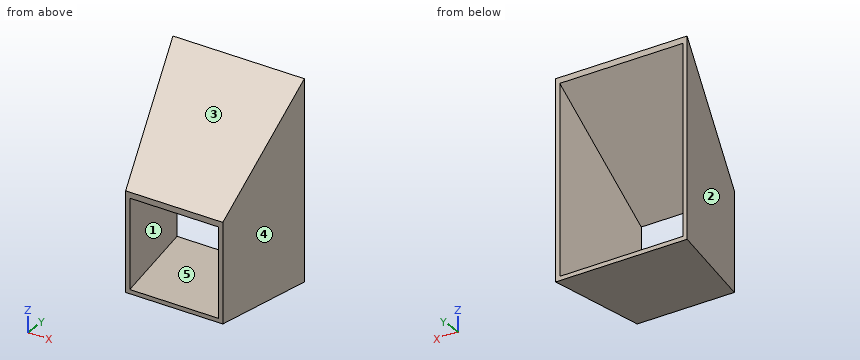
from build123d import *

# Parameters (mm, degrees)
BOSS_EXTRUDE1_DEPTH     = 120
CUT_EXTRUDE1_DEPTH      = 131.179512464
CUT_EXTRUDE1_DEPTH_BACK = 131.179512464
SHELL1_T                = -2.5


with BuildPart() as part:
    # Sketch1 → Boss-Extrude1 (new body)
    with BuildSketch(Plane.XY):
        Polygon((-40.579618843, 30), (40.579618843, 30), (30, -30), (-30, -30), align=None)
    extrude(amount=BOSS_EXTRUDE1_DEPTH)

    # Sketch2 → Cut-Extrude1 (cut, two sides: drawn at the far end of the back side and taken through both)
    with BuildSketch(Plane(origin=(0, 0, 0), x_dir=(0, 0, -1), z_dir=(1, 0, 0)).offset(-CUT_EXTRUDE1_DEPTH_BACK)):
        Polygon((-120, 30), (-120, -30), (-60, -30), align=None)
    extrude(amount=CUT_EXTRUDE1_DEPTH + CUT_EXTRUDE1_DEPTH_BACK, mode=Mode.SUBTRACT)

    # Shell1
    shell1_openings = [part.faces().sort_by_distance(p)[0] for p in [
        (0, -30, 30),
        (0, 30, 60),
    ]]
    offset(amount=SHELL1_T, openings=shell1_openings, kind=Kind.INTERSECTION)


solid = part.part
Part model, mm, in its own coordinate system. Face numbers are marked on the shaded views. A direction names the side the tool comes from. Give positions to 0.01 mm unless a question says otherwise; leave off trailing zeros. Loops run counter-clockwise (first coordinate to the right, second up) from the corner with the lowest first, then second, coordinate; pieces in that order, holes last.
(1) 3-axis set-ups, long thin cutter, end or side, ignore diameter. For the marked faces 1 and 2: which of +Z, -Z, +X, -X, +Y, -Y reach the whole face in a straight line?
Return value:
face 1: +Y
face 2: +Z, -Z, -X, -Y
(2) Drill centre lines: line 1 along Z through (x, y) = (14, -5); line 2 along Z through (x, y) = (-13, -4); line 3 along X through (y, z) = (-12.5, 27). Where is each one in solid material? Low to high.
Return value:
line 1: z = 0 to 2.5, 81.46 to 85
line 2: z = 0 to 2.5, 82.46 to 86
line 3: x = -33.09 to -30.55, 30.55 to 33.09
(3) Pin check, flat tips, straight feed: pin 1 (8 mm diameter, centred on x = -19.5, z = 25, fed in from +Y); pin 2 (1.5 mm diameter, centred on x = 3.5, z = 68, fed in from +Y); pin 3 (4 mm diameter, centred on y = -15, z = 12.5, fed in from -X); pin 4 (1.5 mm diameter, centred on y = 21, z = 38.5, fed in from +X). Stop position of each tip, or through.
Return value:
pin 1: passes through
pin 2: stops at y = -17.71
pin 3: stops at x = -33
pin 4: stops at x = 39.12
(4) Band-saw the part on A-A (x = -0.5). Write the cut outline in (y, z), and give its area (3 significant figures).
Return value:
outline: (-30, 0) - (30, 0) - (30, 2.5) - (-30, 2.5) - close; (-30, 56.46) - (30, 116.46) - (30, 120) - (-30, 60) - close
area: 362 mm2
(5) Band-saw the part on B-B (y = 15). Write the cut outline in (x, z).
Return value:
outline: (-37.93, 0) - (37.93, 0) - (37.93, 105) - (-37.93, 105) - close; hole (-35.4, 2.5) - (35.4, 2.5) - (35.4, 101.46) - (-35.4, 101.46) - close
(6) Pull direction X, two halves, no side cores. Call the marked faces 3, 4 and 5: pulls with the +X half, pulls with the -X half, needs draft (parallel to the pull), parting line crosses it, or undercut.
Return value:
face 3: needs draft
face 4: pulls with the +X half
face 5: undercut
(7) Band-saw the part on C-C (z = 77). Write the cut outline in (x, y).
Return value:
outline: (-40.58, 30) - (-33, -13) - (33, -13) - (40.58, 30) - (38.04, 30) - (31.08, -9.46) - (-31.08, -9.46) - (-38.04, 30) - close
(8) Band-saw the part on D-D (x = -33). Write the cut outline in (y, z).
Return value:
outline: (-12.99, 0) - (30, 0) - (30, 2.5) - (1.41, 2.5) - (1.41, 87.88) - (30, 116.46) - (30, 120) - (-12.99, 77.01) - close
